from build123d import *

# Parameters (mm, degrees)
ESQUISSE2_W             = 24.25
ESQUISSE2_H             = 13.2
ESQUISSE2_R             = 0.5
BOSS_EXTRU_1_DEPTH      = 10.5
ESQUISSE3_W             = 24.25
ESQUISSE3_H             = 13.2
ESQUISSE3_R             = 0.5
ESQUISSE3_R_2           = 2.35
BOSS_EXTRU_2_DEPTH      = 1
ESQUISSE4_W             = 13.55
ESQUISSE4_H             = 5
ENL_V_MAT_EXTRU_1_DEPTH = 30.024343231
CHANFREIN1_SIZE         = 5
BOSS_EXTRU_3_START      = 5.5
BOSS_EXTRU_3_DEPTH      = 5.5
ESQUISSE6_R             = 0.75
ENL_V_MAT_EXTRU_2_DEPTH = 29.540891717
CHANFREIN2_SIZE         = 0.5


with BuildPart() as part:
    # Esquisse2 → Boss.-Extru.1 (new body)
    with BuildSketch(Plane(origin=(0, 0, 0), x_dir=(1, 0, 0), z_dir=(0, 1, 0))):
        with Locations((11.025, 5.5)):
            Rectangle(ESQUISSE2_W, ESQUISSE2_H)
        Polygon((0, 8.5), (2.5, 11), (12.45, 11), (12.45, 0), (2.5, 0), (0, 2.5), align=None, mode=Mode.SUBTRACT)
        with Locations(Location((0.5, 10.5, 0), (0, 0, 270))):
            Circle(ESQUISSE2_R, mode=Mode.SUBTRACT)
        Polygon((19.55, 0), (13.95, 0), (13.95, 11), (19.55, 11), (22.05, 8.5), (22.05, 2.5), align=None, mode=Mode.SUBTRACT)
        with Locations(Location((0.5, 0.5, 0), (0, 0, 270))):
            Circle(ESQUISSE2_R, mode=Mode.SUBTRACT)
        with Locations(Location((21.55, 0.5, 0), (0, 0, 270))):
            Circle(ESQUISSE2_R, mode=Mode.SUBTRACT)
        with Locations(Location((21.55, 10.5, 0), (0, 0, 270))):
            Circle(ESQUISSE2_R, mode=Mode.SUBTRACT)
    extrude(amount=BOSS_EXTRU_1_DEPTH)

    # Esquisse3 → Boss.-Extru.2 (add)
    with BuildSketch(Plane(origin=(0, 10.5, 0), x_dir=(1, 0, 0), z_dir=(0, 1, 0))):
        with Locations((11.025, 5.5)):
            Rectangle(ESQUISSE3_W, ESQUISSE3_H)
        with Locations(Location((0.5, 0.5, 0), (0, 0, 270))):
            Circle(ESQUISSE3_R, mode=Mode.SUBTRACT)
        with Locations(Location((21.55, 0.5, 0), (0, 0, 270))):
            Circle(ESQUISSE3_R, mode=Mode.SUBTRACT)
        with BuildLine():
            ThreePointArc((11.271927083, 5.319972702), (0.725, 5.5), (11.271927083, 5.680027298))
            ThreePointArc((11.271927083, 5.680027298), (12.090678863, 6.244498048), (12.75, 5.5))
            ThreePointArc((12.75, 5.5), (12.090678863, 4.755501952), (11.271927083, 5.319972702))
        make_face(mode=Mode.SUBTRACT)
        with Locations(Location((0.5, 10.5, 0), (0, 0, 270))):
            Circle(ESQUISSE3_R, mode=Mode.SUBTRACT)
        with Locations(Location((18, 5.5, 0), (0, 0, 270))):
            Circle(ESQUISSE3_R_2, mode=Mode.SUBTRACT)
        with Locations(Location((21.55, 10.5, 0), (0, 0, 270))):
            Circle(ESQUISSE3_R, mode=Mode.SUBTRACT)
    extrude(amount=BOSS_EXTRU_2_DEPTH)

    # Esquisse4 → Enlèv. mat.-Extru.1 (cut, through all)
    with BuildSketch(Plane.XY.offset(1.1)):
        with Locations((5.675, 2.5)):
            Rectangle(ESQUISSE4_W, ESQUISSE4_H)
    extrude(amount=-ENL_V_MAT_EXTRU_1_DEPTH, mode=Mode.SUBTRACT)

    # Chanfrein1
    chanfrein1_edges = [part.edges().sort_by_distance(p)[0] for p in [
        (12.45, 5, -11.55),
        (12.45, 5, 0.55),
    ]]
    chamfer(chanfrein1_edges, length=CHANFREIN1_SIZE - 0.0001)  # a hair under: the kernel refuses the full size

    # Esquisse5 → Boss.-Extru.3 (add)
    with BuildSketch(Plane.XZ.offset(-10.5).offset(BOSS_EXTRU_3_START)):
        with BuildLine():
            ThreePointArc((11.79984375, -6.936118893), (13.45, -5.5), (11.79984375, -4.063881107))
            ThreePointArc((11.79984375, -4.063881107), (0.025, -5.5), (11.79984375, -6.936118893))
        make_face()
        with BuildLine():
            ThreePointArc((11.271927083, -5.319972702), (0.725, -5.5), (11.271927083, -5.680027298))
            ThreePointArc((11.271927083, -5.680027298), (12.75, -5.5), (11.271927083, -5.319972702))
        make_face(mode=Mode.SUBTRACT)
    extrude(amount=-BOSS_EXTRU_3_DEPTH)

    # Esquisse6 → Enlèv. mat.-Extru.2 (cut, through all)
    with BuildSketch(Plane(origin=(0, 11.5, 0), x_dir=(1, 0, 0), z_dir=(0, 1, 0))):
        with Locations((12, 5.5)):
            Circle(ESQUISSE6_R)
    extrude(amount=-ENL_V_MAT_EXTRU_2_DEPTH, mode=Mode.SUBTRACT)

    # Chanfrein2
    chanfrein2_edges = [part.edges().sort_by_distance(p)[0] for p in [
        (0.5, 5, -1),
        (0.5, 5, -11),
        (21.55, 0, -1),
        (21.55, 0, -11),
    ]]
    chamfer(chanfrein2_edges, length=CHANFREIN2_SIZE)


solid = part.part
Could you check a few things on this model? Use its own coordinates, in mm. A direction names the side the tool comes from. Give positions to 0.01 mm unless a question says otherwise; leave off trailing zeros. Order: outer loops, then holes, each group sorted by start corner. A loop starts at its lowest first (then second) coordinate and runs counter-clockwise, first axis right, second up.
1. Suppose I cut it at C-C (y = 6.5). State how many separate pieces and enclosed holes the cut face has, plus the area to 3 significant figures.
Answers below:
separate pieces: 1
enclosed holes: 9
area: 125 mm2
2. Suppose I cut it at A-A (x = 6). Write out the boundary of the cut face in (y, z) (3 decimals), plus the area to 3 significant figures.
Answers below:
outline: (5, -12.1) - (11.5, -12.1) - (11.5, -10.775) - (5, -10.775) - close; (5, -0.225) - (11.5, -0.225) - (11.5, 1.1) - (5, 1.1) - close
area: 17.2 mm2
3. Which directions (+Z, -Z, +X, -X, +Y, -Y) give clear straight access to the entire face, cutting with the end or side of a thin tool? Please do faces 4 (the cylindrical face through (0.73, 8.2, -5.27)), 5 (the flat face through (13.95, 5, -5)).
Answers below:
face 4: +Y, -Y
face 5: -Y
4. I need wall thicknesses on L1, parallel to X at y = 4.75, z = -5.5; L2, parallel to Z at x = 0.5, y = 7.55; L3, parallel to X at y = 7.75, z = -3. Which ranges of each line are inside material? Lowest first, please.
Answers below:
L1: x = 12.75 to 13.95, 22.05 to 23.15
L2: z = -12.1 to -11, -10 to -9, -7.83 to -3.17, -2 to -1, 0 to 1.1
L3: x = -1.1 to 0, 0.57 to 1.36, 10.64 to 11.43, 12.45 to 13.95, 22.05 to 23.15
5. Thinking about a two-plate mould opening in Z: for faces 1 (the flat face through (3, 8, 0)), 2 (the flat face through (13, 0, -6)), 3 (the flat face through (14, 7, 1.1)), which applies, +Z half, -Z half, draft (parallel to the pull), parting line (faces both ways), or undercut?
Answers below:
face 1: undercut
face 2: draft
face 3: +Z half
6. Suppose I cut it at B-B (x = 21.55). Write out the boundary of the cut face in (y, z), plus the area to 3 significant figures.
Answers below:
outline: (0, -12.1) - (11.5, -12.1) - (11.5, -11) - (0.5, -11) - (0, -11.5) - close; (0, -9.5) - (0.5, -10) - (11.5, -10) - (11.5, -1) - (0.5, -1) - (0, -1.5) - (0, -2) - (10.5, -2) - (10.5, -9) - (0, -9) - close; (0, 0.5) - (0.5, 0) - (11.5, 0) - (11.5, 1.1) - (0, 1.1) - close
area: 54.8 mm2
7. For pin 1 (3 mm diameter, centred on x = 8, z = -9.5, fed in from +Y); pin 2 (4 mm diameter, centred on x = 19, z = -4.5, fed in from -Y); pin 3 (1.8 mm diameter, centred on x = 2.5, z = -8, fed in from -Y), each with a flat end and sliding along its axis, tell me the tip position at first contact or that it passes through.
Answers below:
pin 1: stops at y = 11.5
pin 2: stops at y = 10.5
pin 3: passes through
